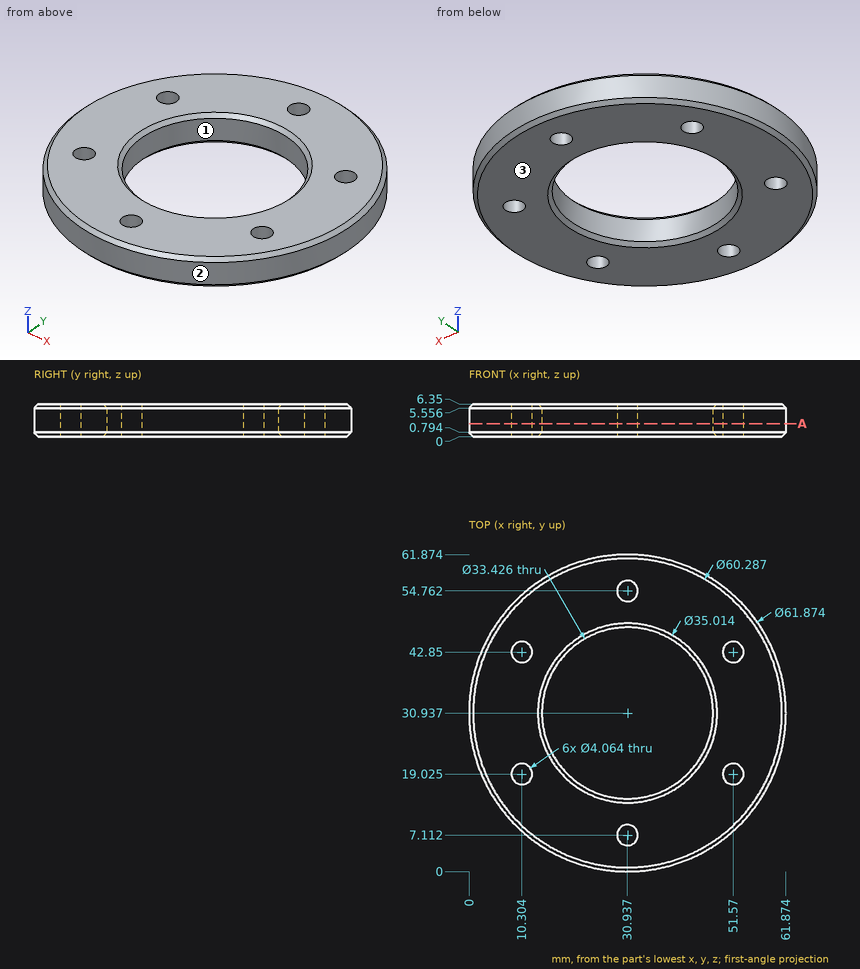
Drawing for the job (mm, zero at the part's lowest x, y, z). Coordinates: 2 decimals unless noted, no trailing zeros. Return JSON: item names as keys, results as strings.
Item 1: Slice it at A-A (z = 2.5). Count the separate pieces of the cut face and the enclosed holes in it, then the cut area to 3 significant figures.
Model answer:
{"separate pieces": "1", "enclosed holes": "7", "area": "2,050 mm²"}
Item 2: Wall check: line 1 along Y through (x, z) = (10.5, 4) (1 decimal); line 2 along Y through (x, z) = (52, 4.5) (1 decimal); line 3 along X through (y, z) = (22, 1) (1 decimal). Give the ranges that are in metal, low to high. Write a range as from..to.
Model answer:
{"line 1": "y = 7.7..17, 21..40.8, 44.9..54.2", "line 2": "y = 8.3..17, 21..40.9, 44.8..53.6", "line 3": "x = 1.3..16.8, 45.1..60.6"}
Item 3: Mould opens along X. For the marked faces 1, 2 and 3 say: pulls with the +X half, pulls with the -X half, needs draft (parallel to the pull), parting line crosses it, or undercut.
Model answer:
{"face 1": "undercut", "face 2": "parting line crosses it", "face 3": "needs draft"}
Item 4: Pin check, flat tips, straight feed: P1, Ø2, axis at x = 51, z = 4, coming from the -Y side; P2, Ø1.5, axis at y = 34.5, z = 5.5, coming from the +X side; P3, Ø1.5, axis at x = 32.5, z = 5.5, coming from the +Y side. Stop position of each tip, or through.
Model answer:
{"P1": "stops at y = 6.57", "P2": "stops at x = 61.75", "P3": "stops at y = 61.86"}
